For this review, take the finished solid that the model builds, in its own axes (mm). Coordinates: 2 decimals unless noted, no trailing zeros. Write each loop counter-clockwise with the first axis right and the second up, starting at its lowest first coordinate (ties: lowest second). Pieces come first, ordered by that corner, then holes.
```python
from build123d import *

# Parameters (mm, degrees)
SKETCH001_R  = 7
POCKET_DEPTH = 4.701


with BuildPart() as part:
    # Sketch → Revolution (revolve)
    with BuildSketch(Plane.XZ):
        Polygon((3, 0), (2.5, 0.288675), (2.5, 4.411325), (3, 4.7), (4.9, 4.7), (6, 4.064915), (6, 0.635085), (4.9, 0), align=None)
    revolve(axis=Axis((0, 0, 0), (0, 0, 1)))

    # Sketch001 → Pocket (cut, through all)
    with BuildSketch(Plane(origin=(0, 0, 4.7), x_dir=(-1, 0, 0), z_dir=(0, 0, 1))):
        with Locations((0.052409, -0.034939)):
            Circle(SKETCH001_R)
        Polygon((5, -2.886751), (5, 2.886751), (0, 5.773503), (-5, 2.886751), (-5, -2.886751), (0, -5.773503), align=None, mode=Mode.SUBTRACT)
    extrude(amount=-POCKET_DEPTH, mode=Mode.SUBTRACT)


solid = part.part
```
Q1. Clearance check with flat-ended pins moving along their axes: pin 1 Ø2 at (x, z) = (-2, 3.5) entering from +Y; pin 2 Ø1.5 at (x, z) = (2.5, 2.5) entering from +Y; pin 3 Ø1 at (x, z) = (3, 2) entering from -Y. State where each tip first meets the part, or that it passes through.
Ans:
pin 1: stops at y = 5.2
pin 2: stops at y = 4.76
pin 3: stops at y = -4.33
Q2. Draft analysis for pull direction Y (two halves, no side actions). For faces 1 (the flat face through (2.535, 4.31, 2.382)), 2 (the cylindrical face through (-0.54, -2.44, 2.38)), 3 (the flat face through (-5, 0, 2)), 4 (the flat face through (-2.535, -4.31, 2.382)), state which applies: +Y half, -Y half, draft (parallel to the pull), parting line (faces both ways), or undercut.
Ans:
face 1: +Y half
face 2: undercut
face 3: draft
face 4: -Y half
Q3. Add section A-A (z = 3.65). State the section outline as (x, y) points.
Ans:
outline: (-5, -2.89) - (0, -5.77) - (5, -2.89) - (5, 2.89) - (0, 5.77) - (-5, 2.89) - close; hole circle Ø5 at (0, 0)
Q4. Add section B-B (y = 0). State the section outline as (x, z) points, then the cut area to 3 significant figures.
Ans:
outline: (-5, 0.06) - (-4.9, 0) - (-3, 0) - (-2.5, 0.29) - (-2.5, 4.41) - (-3, 4.7) - (-4.9, 4.7) - (-5, 4.64) - close; (2.5, 0.29) - (3, 0) - (4.9, 0) - (5, 0.06) - (5, 4.64) - (4.9, 4.7) - (3, 4.7) - (2.5, 4.41) - close
area: 23.2 mm2
Q5. For probe 1 along Y at (x, z) = (-1, 2.35); probe 2 along X at (y, z) = (-0.25, 1.35); probe 3 along Y at (x, z) = (-4, 3.8), list the stretches that pass through material, from the lowest coordinate up.
Ans:
probe 1: y = -5.2 to -2.29, 2.29 to 5.2
probe 2: x = -5 to -2.49, 2.49 to 5
probe 3: y = -3.46 to 3.46
